Geometry: final body of the model. Coordinates: model frame, mm. Face numbers are marked on the shaded views. A direction names the side the tool comes from. Round coordinates to 2 decimals unless told otherwise and drop trailing zeros. Order: outer loops, then holes, each group sorted by start corner. A loop starts at its lowest first (then second) coordinate and runs counter-clockwise, first axis right, second up. Notation, with made-up numbers: (-37, 83.25) -> (-9, 83.25) arc R18 ccw to (-9, 98.25) -> close; hole circle Ø10 at (-22, 50). An arc over 180 degrees is marked (long way). Put each result on its own line as item: value.
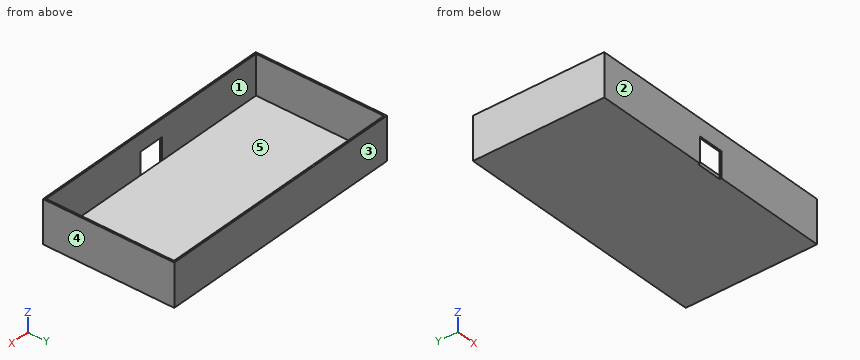
```python
from build123d import *

# Parameters (mm, degrees)
F0_W     = 149
F0_H     = 77
F1_DEPTH = 25
F2_W     = 147
F2_H     = 75
F3_DEPTH = 23
F4_W     = 15
F4_H     = 15
F5_DEPTH = 1


with BuildPart() as f1:
    # F0 (on Top) → F1 (new body)
    with BuildSketch(Plane.XY):
        Rectangle(F0_W, F0_H)
    extrude(amount=F1_DEPTH)

    # F2 (on face) → F3 (cut)
    with BuildSketch(Plane.XY.offset(25)):
        Rectangle(F2_W, F2_H)
    extrude(amount=-F3_DEPTH, mode=Mode.SUBTRACT)

    # F4 (on face) → F5 (cut)
    with BuildSketch(Plane.XZ.offset(38.5)):
        with Locations((0, 7.5)):
            Rectangle(F4_W, F4_H)
    extrude(amount=-F5_DEPTH, mode=Mode.SUBTRACT)


solid = f1.part
```
1. Material intervals for probe 1 along X at (y, z) = (31, 17.75); probe 2 along Y at (x, z) = (-66.5, 20.5); probe 3 along Z at (x, y) = (-53.5, 5.5), sorted ascending.
Ans:
probe 1: -74.5 to -73.5, 73.5 to 74.5
probe 2: -38.5 to -37.5, 37.5 to 38.5
probe 3: 0 to 2
2. Draft query along Y for the marked faces 3, 4 and 5. Return one class per face: +Y half, -Y half, draft (parallel to the pull), parting line (faces both ways), or undercut.
Ans:
face 3: +Y half
face 4: draft
face 5: undercut
3. Cut plane A-A on z = 22.75. Return loops of the section in (x, y).
Ans:
outline: (-74.5, -38.5) -> (74.5, -38.5) -> (74.5, 38.5) -> (-74.5, 38.5) -> close; hole (-73.5, -37.5) -> (73.5, -37.5) -> (73.5, 37.5) -> (-73.5, 37.5) -> close
4. Cut plane D-D on y = -3. Return loops of the section in (x, z).
Ans:
outline: (-74.5, 0) -> (74.5, 0) -> (74.5, 25) -> (73.5, 25) -> (73.5, 2) -> (-73.5, 2) -> (-73.5, 25) -> (-74.5, 25) -> close
5. Contact query for a flat-ended pin moving along its axis: P1, Ø1.6, axis at x = 3, z = 0.5, coming from the -Y side. Output: stop coordinate, or through.
Ans:
P1: y = -37.5
6. Cut plane C-C on z = 12.25. Return loops of the section in (x, y), and give its area (3 significant figures).
Ans:
outline: (-74.5, -38.5) -> (-7.5, -38.5) -> (-7.5, -37.5) -> (-73.5, -37.5) -> (-73.5, 37.5) -> (73.5, 37.5) -> (73.5, -37.5) -> (7.5, -37.5) -> (7.5, -38.5) -> (74.5, -38.5) -> (74.5, 38.5) -> (-74.5, 38.5) -> close
area: 433 mm²
7. Cut plane B-B on x = 24.5. Return loops of the section in (y, z), and give its area (3 significant figures).
Ans:
outline: (-38.5, 0) -> (38.5, 0) -> (38.5, 25) -> (37.5, 25) -> (37.5, 2) -> (-37.5, 2) -> (-37.5, 25) -> (-38.5, 25) -> close
area: 200 mm²
8. Set-up query: the marked faces 1 and 2. Return all of +Z, -Z, +X, -X, +Y, -Y with unobstructed straight access to the full face (end or side cutting, diameter ignored); none if empty.
Ans:
face 1: +Z
face 2: +Z, -Z, +X, -X, -Y
